Input: part model. Units: mm. Frame: model coordinates. A direction names the side the tool comes from. Round coordinates to 2 decimals unless told otherwise and drop trailing zeros. Write each loop counter-clockwise with the first axis right and the second up, starting at its lowest first coordinate (ties: lowest second). Pieces come first, ordered by that corner, then holes. Notation, with made-up numbers: M -30.75,10 L -19.75,10 A17 cw -19.75,20 Z; hole C 72,1 d2. An arc over 180 degrees is marked long. Write each question's results on one line, items separated by ' | '. Start each with the question number.
```python
from build123d import *

# Parameters (mm, degrees)
SKETCH_1_R          = 22.5
EXTRUDE_1_DEPTH     = 8
SKETCH_2_R          = 40
EXTRUDE_2_DEPTH     = 3
SKETCH_4_R          = 19.5
CUT_EXTRUDE_2_DEPTH = 58.628118137
SKETCH_7_R          = 1.25
CUT_EXTRUDE_4_DEPTH = 58.628118137


with BuildPart() as part:
    # 草图1 → 凸台-拉伸1 (new body)
    with BuildSketch(Plane.XY):
        Circle(SKETCH_1_R)
    extrude(amount=EXTRUDE_1_DEPTH)

    # 草图2 → 凸台-拉伸2 (add)
    with BuildSketch(Plane(origin=(0, 0, 0), x_dir=(-1, 0, 0), z_dir=(0, 0, -1))):
        Circle(SKETCH_2_R)
    extrude(amount=EXTRUDE_2_DEPTH)

    # 草图4 → 切除-拉伸2 (cut, through all)
    with BuildSketch(Plane.XY.offset(8)):
        Circle(SKETCH_4_R)
    extrude(amount=-CUT_EXTRUDE_2_DEPTH, mode=Mode.SUBTRACT)

    # 草图7 → 切除-拉伸4 (cut, through all)
    with BuildSketch(Plane(origin=(0, 0, -3), x_dir=(-1, 0, 0), z_dir=(0, 0, -1))):
        with Locations((32.5, 19.691368668)):
            Circle(SKETCH_7_R)
        with Locations((-32.5, 19.691368668)):
            Circle(SKETCH_7_R)
        with Locations((32.5, -19.691368668)):
            Circle(SKETCH_7_R)
        with Locations((-32.5, -19.691368668)):
            Circle(SKETCH_7_R)
    extrude(amount=-CUT_EXTRUDE_4_DEPTH, mode=Mode.SUBTRACT)


solid = part.part
```
1. Draft query along X for faces 3 (the face through (8.67, -39.05, -1.48)), 4 (the face through (-17, -17, 0)), 5 (the face through (-2.539, 19.334, 2.577)). Return one class per face: +X half, -X half, draft (parallel to the pull), parting line (faces both ways), or undercut.
2. Access query for faces 1 (the face through (-33.077, 18.582, -1.521)), 2 (the face through (10.382, -19.961, 3.944)). Directions: +Z, -Z, +X, -X, +Y, -Y. A direction counts if a zero-diameter tool reaches every point of the face in a straight line with its end or side. Return the directions, or none.
3. Contact query for flat-ended pins moving along their axis: P1, Ø4, axis at x = -32.5, y = 19.69, coming from the +Z side; P2, Ø4, axis at y = 17.5, z = 3.5, coming from the +X side; P3, Ø1.5, axis at y = 8.5, z = 7, coming from the -X side; P4, Ø1.5, axis at y = -24.5, z = 6.5, coming from the +X side. Output: stop coordinate, or through.
4. Cut plane A-A on y = 0. Output: boundary loops of the cut face in (x, z).
5. Cut plane C-C on z = 3.75. Output: boundary loops of the cut face in (x, y).
6. Line query: L1, parallel to Y at x = -32.5, z = -2.25; L2, parallel to Y at x = 0, z = 4.25; L3, parallel to Z at x = -33, y = 14. Output: solid intervals per line, ascending. Write a range as from..to.
7. Cut plane D-D on x = -32.5. Output: boundary loops of the cut face in (y, z).
Answers follow:
1) face 3: parting line | face 4: draft | face 5: undercut
2) face 1: +Z, -Z | face 2: +Z
3) P1: stops at z = 0 | P2: stops at x = 16.31 | P3: stops at x = -21.12 | P4: passes through
4) outline: M -40,-3 L -19.5,-3 L -19.5,8 L -22.5,8 L -22.5,0 L -40,0 Z; M 19.5,-3 L 40,-3 L 40,0 L 22.5,0 L 22.5,8 L 19.5,8 Z
5) outline: C 0,0 d45; hole C 0,0 d39
6) L1: y = -23.32..-20.94, -18.44..18.44, 20.94..23.32 | L2: y = -22.5..-19.5, 19.5..22.5 | L3: z = -3..0
7) outline: M -23.32,-3 L -20.94,-3 L -20.94,0 L -23.32,0 Z; M -18.44,-3 L 18.44,-3 L 18.44,0 L -18.44,0 Z; M 20.94,-3 L 23.32,-3 L 23.32,0 L 20.94,0 Z
